Geometry check sheet. Reference: the model listing, model coordinates, mm. A direction names the side the tool comes from. Give positions to 0.01 mm unless a question says otherwise; leave off trailing zeros. Write each loop counter-clockwise with the first axis right and the second up, starting at its lowest first coordinate (ties: lowest second). Pieces come first, ordered by that corner, then holes.
(1) Cross-section at A-A (y = 2). Record the boundary of the cut face in (x, z), and give its area (3 significant figures).
(2) Depth check by flat-ended pin: P1, Ø1.9, axis at x = 6.5, z = 100, coming from the -Y side. Enter the tip coordinate at first touch or a pass-through.
(3) Cross-section at C-C (x = 6.5). Record the boundary of the cut face in (y, z), and give its area (3 significant figures).
(4) Thickness scan on line 1 along X through (y, z) = (-0.3, 10); line 2 along Y through (x, z) = (9.5, 46). Record the ranges inside material, lowest first.
(5) Cross-section at B-B (z = 54). Record the boundary of the cut face in (x, y), and give its area (3 significant figures).
(6) Tool access check on faces 4 (the flat face through (6, -1, 54)), 5 (the flat face through (6, 13, 54)). Record the directions out of +Z, -Z, +X, -X, +Y, -Y that give a thin tool (end or side, any length) a straight path to the whole face; none if there is none.
(7) Mould release check, pull along Z, two halves, no side actions. Record for faces 1 (the flat face through (-0.3, 6.6, 0)), 2 (the flat face through (6, 14, 54)), 3 (the cylindrical face through (5.53, 13.51, 8.73)): +Z half, -Z half, draft (parallel to the pull), parting line (faces both ways), or undercut.
(8) Cross-section at D-D (z = 100). Record the boundary of the cut face in (x, y).
```python
from build123d import *

# Parameters (mm, degrees)
SKETCH_1_W          = 15
SKETCH_1_H          = 15
SKETCH_1_W_2        = 13
SKETCH_1_H_2        = 13
EXTRUDE_1_DEPTH     = 110
SKETCH_2_R          = 1.6
CUT_EXTRUDE_1_DEPTH = 32


with BuildPart() as part:
    # 草图1 → 拉伸-薄壁1 (new body)
    with BuildSketch(Plane.XY):
        with Locations((6.5, 6.5)):
            Rectangle(SKETCH_1_W, SKETCH_1_H)
        with Locations((6.5, 6.5)):
            Rectangle(SKETCH_1_W_2, SKETCH_1_H_2, mode=Mode.SUBTRACT)
    extrude(amount=EXTRUDE_1_DEPTH)

    # 草图2 → 切除-拉伸1 (cut)
    with BuildSketch(Plane(origin=(0, 14, 0), x_dir=(1, 0, 0), z_dir=(0, 1, 0))):
        with Locations(Location((6.5, -10, 0), (0, 0, 270))):
            Circle(SKETCH_2_R)
        with Locations(Location((6.5, -100, 0), (0, 0, 270))):
            Circle(SKETCH_2_R)
    extrude(amount=-CUT_EXTRUDE_1_DEPTH, mode=Mode.SUBTRACT)


solid = part.part
```
Reply:
1. outline: (-1, 0) - (0, 0) - (0, 110) - (-1, 110) - close; (13, 0) - (14, 0) - (14, 110) - (13, 110) - close
1. area: 220 mm2
2. P1: passes through
3. outline: (-1, 0) - (0, 0) - (0, 8.4) - (-1, 8.4) - close; (-1, 11.6) - (0, 11.6) - (0, 98.4) - (-1, 98.4) - close; (-1, 101.6) - (0, 101.6) - (0, 110) - (-1, 110) - close; (13, 0) - (14, 0) - (14, 8.4) - (13, 8.4) - close; (13, 11.6) - (14, 11.6) - (14, 98.4) - (13, 98.4) - close; (13, 101.6) - (14, 101.6) - (14, 110) - (13, 110) - close
3. area: 207 mm2
4. line 1: x = -1 to 4.9, 8.1 to 14
4. line 2: y = -1 to 0, 13 to 14
5. outline: (-1, -1) - (14, -1) - (14, 14) - (-1, 14) - close; hole (0, 0) - (13, 0) - (13, 13) - (0, 13) - close
5. area: 56.0 mm2
6. face 4: +Z, -Z, +X, -X, -Y
6. face 5: +Z, -Z
7. face 1: -Z half
7. face 2: draft
7. face 3: undercut
8. outline: (-1, -1) - (4.9, -1) - (4.9, 0) - (0, 0) - (0, 13) - (4.9, 13) - (4.9, 14) - (-1, 14) - close; (8.1, -1) - (14, -1) - (14, 14) - (8.1, 14) - (8.1, 13) - (13, 13) - (13, 0) - (8.1, 0) - close
